```python
from build123d import *

# Parameters (mm, degrees)
F0_W     = 29
F0_H     = 50
F3_D     = 2
F3_DEPTH = 3
F3_TIP   = 0.600860619
F4_R     = 1
F5_R     = 6
F6_DEPTH = 5


with BuildPart() as f2:
    # F2: sweep along a path in F1
    with BuildLine(Plane.XZ) as f2_path:
        Line((0, 0), (0, 14))
    # F0 (on Top) → F2 (sweep)
    with BuildSketch(Plane.XY):
        Rectangle(F0_W, F0_H)
    sweep(path=f2_path.line)

    # F3
    with Locations(Plane(origin=(0, 0, 0), x_dir=(1, 0, 0), z_dir=(0, 0, -1))):
        with Locations((5, -5), (-5, -5), (-5, 5), (5, 5)):
            Hole(F3_D / 2, depth=F3_DEPTH)
            with Locations((0, 0, -(F3_DEPTH + F3_TIP / 2))):  # 118° drill point
                Cone(0, F3_D / 2, F3_TIP, mode=Mode.SUBTRACT)

    # F4
    f4_edges = [f2.edges().sort_by_distance(p)[0] for p in [
        (14.5, -25, 7),
        (-14.5, -25, 7),
        (14.5, 25, 7),
        (-14.5, 25, 7),
    ]]
    fillet(f4_edges, radius=F4_R)

    # F5 (on face) → F6 (join)
    with BuildSketch(Plane(origin=(0, 25, 0), x_dir=(-1, 0, 0), z_dir=(0, 1, 0))):
        with Locations((0, 6.833284162)):
            Circle(F5_R)
    extrude(amount=F6_DEPTH)


solid = f2.part
```
Check sheet for the modelled part. Datum: model origin and axes. Units: mm. A direction names the side the tool comes from. Coordinates: 2 decimals unless noted, no trailing zeros. Loops run counter-clockwise (first coordinate to the right, second up) from the corner with the lowest first, then second, coordinate; pieces in that order, holes last.
1) Material ranges on probe 1 along X at (y, z) = (5, 0.75); probe 2 along Y at (x, z) = (-5, 1.45); probe 3 along Y at (x, z) = (-10.75, 9.25), recorded low to high.
2) Access from +Z, -Z, +X, -X, +Y, -Y to the whole of each face (thin tool, end or side, straight path). Record for faces 4 (the face through (1.301, 27.465, 0.976)), 5 (the face through (-5, 4, 2)), 6 (the face through (0, 0, 14)).
3) Gauge pin test, flat ends, axial feed: pin 1 (1 mm diameter, centred on x = 8, z = 9.5, fed in from +Y); pin 2 (1.6 mm diameter, centred on x = -5, y = 5, fed in from -Z). Record the tip position at first contact, or that the pin passes through.
4) Sectioned sample at B-B (x = 8.5). Record the boundary of the cut face in (y, z), and give its area (3 significant figures).
5) Sectioned sample at A-A (z = 1.75). Record the boundary of the cut face in (x, y).
6) Release check for a two-part mould opening along X. For faces 1 (the face through (5, 4, 2)), 2 (the face through (14.199, 24.715, 7.098)), 3 (the face through (0, -25, 7)) record: released by +X, released by -X, zero draft, split by the parting line, or undercut.
Check sheet entries:
1. probe 1: x = -14.5 to -6, -4 to 4, 6 to 14.5
1. probe 2: y = -25 to -6, -4 to 4, 6 to 25
1. probe 3: y = -25 to 25
2. face 4: +Y
2. face 5: -Z
2. face 6: +Z, +X, -X, +Y, -Y
3. pin 1: stops at y = 25
3. pin 2: stops at z = 3.12
4. outline: (-25, 0) - (25, 0) - (25, 14) - (-25, 14) - close
4. area: 700 mm2
5. outline: (-14.5, -24) arc R1 ccw to (-13.5, -25) - (13.5, -25) arc R1 ccw to (14.5, -24) - (14.5, 24) arc R1 ccw to (13.5, 25) - (3.19, 25) - (3.19, 30) - (-3.19, 30) - (-3.19, 25) - (-13.5, 25) arc R1 ccw to (-14.5, 24) - close; hole circle Ø2 at (-5, -5); hole circle Ø2 at (-5, 5); hole circle Ø2 at (5, -5); hole circle Ø2 at (5, 5)
6. face 1: undercut
6. face 2: released by +X
6. face 3: zero draft
